Design review of the part built by this model. Coordinates are the model's own, in mm. Face numbers are marked on the shaded views. A direction names the side the tool comes from. Round coordinates to 2 decimals unless told otherwise and drop trailing zeros. Loops run counter-clockwise (first coordinate to the right, second up) from the corner with the lowest first, then second, coordinate; pieces in that order, holes last. Notation, with made-up numbers: M -39,18 L 0,18 A24 ccw 0,38 Z; hole C 12.25,86.5 d7. An arc over 180 degrees is marked long. Use a Markdown table: item, result.
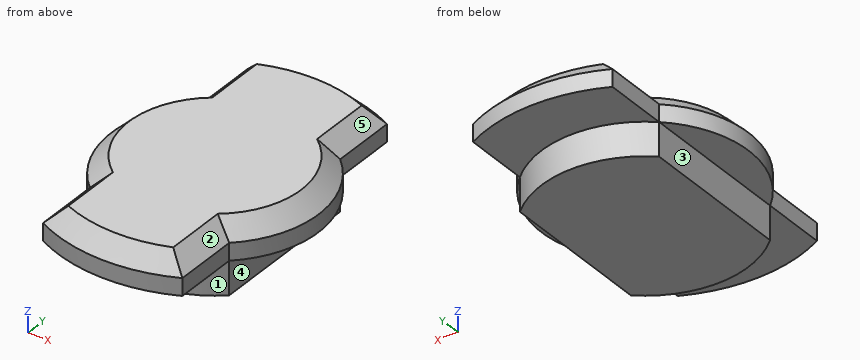
from build123d import *

# Parameters (mm, degrees)
PAD007_DEPTH = 1.6
CHAMFER_SIZE = 0.8
PAD008_DEPTH = 1.55


with BuildPart() as part:
    # Sketch011 → Pad007 (new body)
    with BuildSketch(Plane.XY):
        with BuildLine():
            Line((-3.230712, 3.55), (-3.230712, 6.546182))
            ThreePointArc((3.230712, 6.546182), (0, 7.3), (-3.230712, 6.546182))
            Line((3.230712, 3.55), (3.230712, 6.546182))
            ThreePointArc((3.230712, -3.55), (4.8, 0), (3.230712, 3.55))
            Line((3.230712, -3.55), (3.230712, -6.546182))
            ThreePointArc((-3.230712, -6.546182), (0, -7.3), (3.230712, -6.546182))
            Line((-3.230712, -3.55), (-3.230712, -6.546182))
            ThreePointArc((-3.230712, 3.55), (-4.8, 0), (-3.230712, -3.55))
        make_face()
    extrude(amount=PAD007_DEPTH)

    # Chamfer
    chamfer_edges = [part.edges().sort_by_distance(p)[0] for p in [
        (-4.8, 0, 1.6),
        (-3.230712, -5.048091, 1.6),
        (0, -7.3, 1.6),
        (3.230712, -5.048091, 1.6),
        (4.8, 0, 1.6),
        (3.230712, 5.048091, 1.6),
        (0, 7.3, 1.6),
        (-3.230712, 5.048091, 1.6),
    ]]
    chamfer(chamfer_edges, length=CHAMFER_SIZE)

    # Sketch013 (on Face4 of Chamfer) → Pad008 (join)
    with BuildSketch(Plane(origin=(0, 0, 0), x_dir=(1, 0, 0), z_dir=(0, 0, -1))):
        with BuildLine():
            Line((-3.230712, 3.55), (-3.230712, -3.55))
            ThreePointArc((-3.230712, -3.55), (0, -4.8), (3.230712, -3.55))
            Line((3.230712, 3.55), (3.230712, -3.55))
            ThreePointArc((3.230712, 3.55), (0, 4.8), (-3.230712, 3.55))
        make_face()
    extrude(amount=PAD008_DEPTH)


with BuildPart() as part_1:
    # Body002 placement: moved
    add(part.part.moved(Location((0, 0, 0.8))))


solid = part_1.part
1. Take a section at A-A on z = 1.15. Give the boundary of the cut face in (x, y).
Check values:
| item | result |
|---|---|
| outline | M -3.23,-6.55 A7.3 ccw 3.23,-6.55 L 3.23,-3.55 A4.8 ccw 3.23,3.55 L 3.23,6.55 A7.3 ccw -3.23,6.55 L -3.23,3.55 A4.8 ccw -3.23,-3.55 Z |
2. Machinability: for the marked faces 1, 2, 3, 4 and 5, which of the approach directions +Z, -Z, +X, -X, +Y, -Y give a long, thin tool a straight path to every point of the face, cutting with its end or side? Answer none if there is none.
Check values:
| item | result |
|---|---|
| face 1 | -Z, -Y |
| face 2 | +Z, +X, -Y |
| face 3 | -Z, -X, +Y, -Y |
| face 4 | -Z, +X, +Y, -Y |
| face 5 | +Z, +X, +Y |
3. Take a section at C-C on z = -0.1. Give the boundary of the cut face in (x, y), and give its area (3 significant figures).
Check values:
| item | result |
|---|---|
| outline | M -3.23,-3.55 A4.8 ccw 3.23,-3.55 L 3.23,3.55 A4.8 ccw -3.23,3.55 Z |
| area | 57.0 mm² |
4. Take a section at B-B on y = 4.5. Give the boundary of the cut face in (x, z), and give its area (3 significant figures).
Check values:
| item | result |
|---|---|
| outline | M -3.23,0.8 L -1.67,0.8 L -1.67,-0.75 L 1.67,-0.75 L 1.67,0.8 L 3.23,0.8 L 3.23,1.6 L 2.43,2.4 L -2.43,2.4 L -3.23,1.6 Z |
| area | 14.9 mm² |
5. Take a section at D-D on z = 1.8. Give the boundary of the cut face in (x, y), and give its area (3 significant figures).
Check values:
| item | result |
|---|---|
| outline | M -3.03,-6.42 A7.1 ccw 3.03,-6.42 L 3.03,-3.46 A4.6 ccw 3.03,3.46 L 3.03,6.42 A7.1 ccw -3.03,6.42 L -3.03,3.46 A4.6 ccw -3.03,-3.46 Z |
| area | 98.4 mm² |
6. Wall thickness on line 1 along X through (y, z) = (-4, 0.95); line 2 along Z through (x, y) = (1.5, -4.75); line 3 along Z through (x, y) = (2, 6.75): over which ranges is each line inside the solid? List them lowest first. Write a range as from..to.
Check values:
| item | result |
|---|---|
| line 1 | x = -3.23..3.23 |
| line 2 | z = 0.8..2.4 |
| line 3 | z = 0.8..1.86 |
7. Insertion check: pin 1 (1.2 mm diameter, centred on y = 0, z = 0, fed in from +X); pin 2 (0.5 mm diameter, centred on y = -0.5, z = 0, fed in from -X); pin 3 (1.9 mm diameter, centred on x = -1.5, y = -6, fed in from -Z). Each pin has a flat end and moves straight along its axis. Give the tip position at first contact, or say it passes through.
Check values:
| item | result |
|---|---|
| pin 1 | stops at x = 3.23 |
| pin 2 | stops at x = -3.23 |
| pin 3 | stops at z = 0.8 |
